```python
from build123d import *

# Parameters (mm, degrees)
SKETCH1_W           = 60
SKETCH1_H           = 20
BOSS_EXTRUDE1_DEPTH = 2.5
SKETCH2_W           = 20
SKETCH2_H           = 1.66
CUT_EXTRUDE1_DEPTH  = 37.142080737


with BuildPart() as part:
    # Sketch1 → Boss-Extrude1 (new, symmetric)
    with BuildSketch(Plane.XY):
        Rectangle(SKETCH1_W, SKETCH1_H)
    extrude(amount=BOSS_EXTRUDE1_DEPTH, both=True)

    # Sketch2 → Cut-Extrude1 (cut, through all)
    with BuildSketch(Plane(origin=(0, 10, 0), x_dir=(1, 0, 0), z_dir=(0, 1, 0))):
        with Locations((-20, 0)):
            Rectangle(SKETCH2_W, SKETCH2_H)
        with Locations((20, 1.67)):
            Rectangle(SKETCH2_W, SKETCH2_H)
        with Locations((20, -1.67)):
            Rectangle(SKETCH2_W, SKETCH2_H)
    extrude(amount=-CUT_EXTRUDE1_DEPTH, mode=Mode.SUBTRACT)


solid = part.part
```
Input: part model. Units: mm. Frame: model coordinates. A direction names the side the tool comes from. Coordinates: 2 decimals unless noted, no trailing zeros. Write each loop counter-clockwise with the first axis right and the second up, starting at its lowest first coordinate (ties: lowest second). Pieces come first, ordered by that corner, then holes.
1) Pin query (flat end, axial travel): pin 1 Ø4 at (x, y) = (14.5, 1) entering from +Z; pin 2 Ø0.5 at (y, z) = (-4.5, 1.5) entering from +X; pin 3 Ø0.5 at (y, z) = (-2, -0.5) entering from -X. Return the tip coordinate at first contact, or that it passes through.
2) Mould query, pull axis Z, two halves, no side actions, for faces 4 (the flat face through (-10, 0, 2.5)), 5 (the flat face through (-20, 0, -0.83)), 6 (the flat face through (20, 0, -0.84)). Classes: pulls with the +Z half, pulls with the -Z half, needs draft (parallel to the pull), parting line crosses it, or undercut.
3) Section C-C on x = 23.5. Output: boundary loops of the cut face in (y, z), and give its area (3 significant figures).
4) Section B-B on y = -1.25. Output: boundary loops of the cut face in (x, z), and give its area (3 significant figures).
5) Set-up query: faces 1 (the flat face through (-10, 0, 0)), 2 (the flat face through (10, 0, -2)), 3 (the flat face through (10, 0, 2)). Return all of +Z, -Z, +X, -X, +Y, -Y with unobstructed straight access to the full face (end or side cutting, diameter ignored); none if empty.
6) Material intervals for line 1 along Z through (x, y) = (-19, 2); line 2 along X through (y, z) = (9.25, 2.1); line 3 along X through (y, z) = (-5.5, 0), sorted ascending.
7) Section A-A on x = -19.5. Output: boundary loops of the cut face in (y, z), and give its area (3 significant figures).
8) Section D-D on z = -1.45. Output: boundary loops of the cut face in (x, y), and give its area (3 significant figures).
Check result:
1. pin 1: stops at z = 0.84
1. pin 2: stops at x = 10
1. pin 3: stops at x = -10
2. face 4: pulls with the +Z half
2. face 5: undercut
2. face 6: pulls with the -Z half
3. outline: (-10, -0.84) - (10, -0.84) - (10, 0.84) - (-10, 0.84) - close
3. area: 33.6 mm2
4. outline: (-30, -2.5) - (10, -2.5) - (10, -0.84) - (30, -0.84) - (30, 0.84) - (10, 0.84) - (10, 2.5) - (-30, 2.5) - (-30, 0.83) - (-10, 0.83) - (-10, -0.83) - (-30, -0.83) - close
4. area: 200 mm2
5. face 1: -X, +Y, -Y
5. face 2: -Z, +X, +Y, -Y
5. face 3: +Z, +X, +Y, -Y
6. line 1: z = -2.5 to -0.83, 0.83 to 2.5
6. line 2: x = -30 to 10
6. line 3: x = -10 to 30
7. outline: (-10, -2.5) - (10, -2.5) - (10, -0.83) - (-10, -0.83) - close; (-10, 0.83) - (10, 0.83) - (10, 2.5) - (-10, 2.5) - close
7. area: 66.8 mm2
8. outline: (-30, -10) - (10, -10) - (10, 10) - (-30, 10) - close
8. area: 800 mm2
